Geometry: see drawing. Coordinates: mm, zero at the bounding-box minimum. A direction names the side the tool comes from. Coordinates: 2 decimals unless noted, no trailing zeros. Order: outer loops, then holes, each group sorted by start corner. A loop starts at its lowest first (then second) coordinate and runs counter-clockwise, first axis right, second up. Notation, with made-up numbers: M 21,-3.5 L 30,-3.5 A4 cw 30,1.5 Z; hole C -38,19.25 d10. An arc over 180 degrees is marked long. One line per item, written item: value.
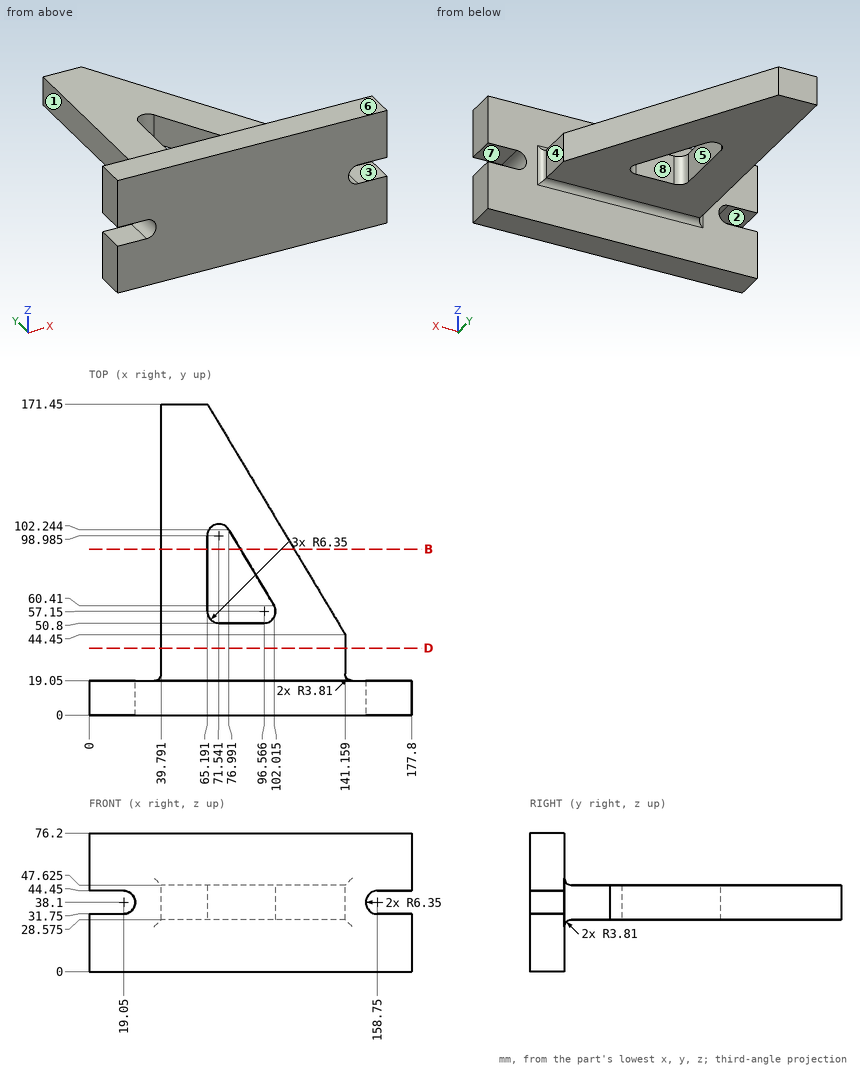
(1) Draft query along Z for the marked faces 6, 7 and 8. Return one class per face: released by +Z, released by -Z, zero draft, split by the parting line, or undercut.
Data:
face 6: released by +Z
face 7: undercut
face 8: zero draft
(2) Access query for the marked faces 1, 2, 3, 4 and 5. Directions: +Z, -Z, +X, -X, +Y, -Y. A direction counts if a zero-diameter tool reaches every point of the face in a straight line with its end or side. Return the directions, or none.
Data:
face 1: +Z, -Z, -X, +Y
face 2: -X, +Y, -Y
face 3: +X, +Y, -Y
face 4: +Z, -Z, +X, +Y
face 5: +Z, -Z
(3) First-contact query: pin 1 (1 mm diameter, centred on x = 42, z = 17, fed in from +Y); pin 2 (4 mm diameter, centred on y = 119.5, z = 45.5, fed in from +X); pin 3 (5.5 mm diameter, centred on x = 173, y = 5.5, fed in from -Z); pin 4 (15 mm diameter, centred on y = 34.5, z = 37, fed in from +X). Flat tips, straight axial feed; report the tip coordinate or a pass-through.
Data:
pin 1: stops at y = 19.05
pin 2: stops at x = 97.46
pin 3: stops at z = 0
pin 4: stops at x = 141.16
(4) Cut plane D-D on y = 37. Output: boundary loops of the cut face in (x, z) (1 decimal), plus the area to 3 significant figures.
Data:
outline: M 39.8,28.6 L 141.2,28.6 L 141.2,47.6 L 39.8,47.6 Z
area: 1,930 mm2
(5) Ray query, line 1 (Y direction, x = 149, z = 22.5); line 2 (Z direction, x = 55, y = 70) (1 decimal); line 3 (Z direction, x = 16, y = 15). Return the intervals inside material, ascending. Write a range as from..to.
Data:
line 1: y = 0..19.05
line 2: z = 28.6..47.6
line 3: z = 0..31.75, 44.45..76.2
(6) Cut plane B-B on y = 91.5. Output: boundary loops of the cut face in (x, z) (1 decimal).
Data:
outline: M 39.8,28.6 L 65.2,28.6 L 65.2,47.6 L 39.8,47.6 Z; M 83.4,28.6 L 113,28.6 L 113,47.6 L 83.4,47.6 Z
